Here's the drawing with two shaded views (mm, measured from the low corner). I have some questions. Round coordinates to 2 decimals unless told otherwise and drop trailing zeros. Loops run counter-clockwise (first coordinate to the right, second up) from the corner with the lowest first, then second, coordinate; pieces in that order, holes last.
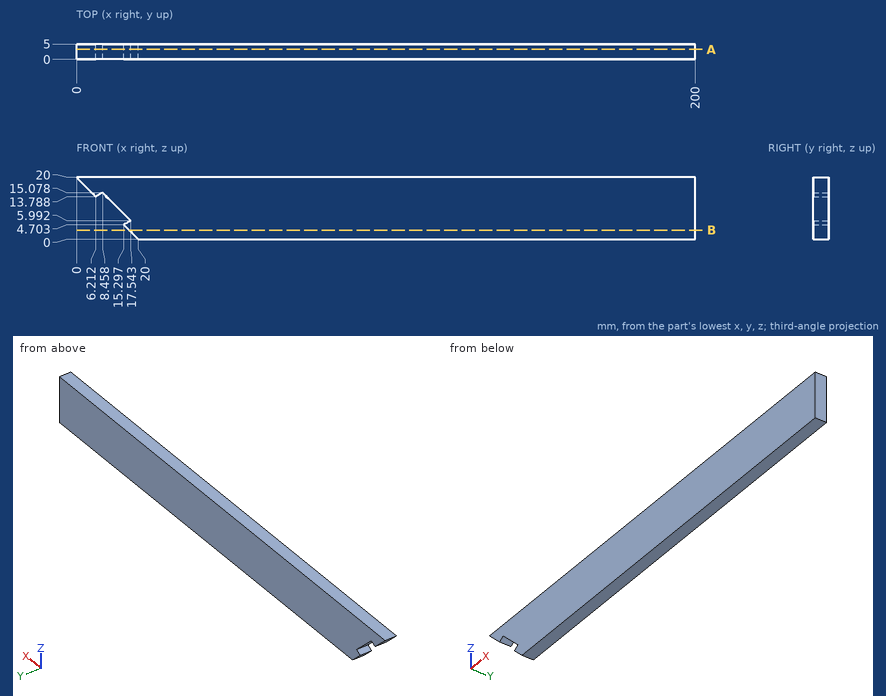
(1) If I drill on line 1 (Z direction, x = 9.5, y = 1.85) (1 decimal); line 2 (X direction, y = 4.3, z = 16.25); line 3 (X direction, y = 2.6, z = 2), over which ranges is the centre line in solid material (lowest first)?
Worked answers:
line 1: z = 14 to 20
line 2: x = 3.75 to 200
line 3: x = 18 to 200
(2) If we section it at B-B, the plane z = 3: List the corners of the cut face in (x, y) for me, then the cut area to 3 significant figures.
Worked answers:
outline: (17, 0) - (200, 0) - (200, 5) - (17, 5) - close
area: 915 mm2
(3) If we section it at A-A, the plane y = 3.25: List the corners of the cut face in (x, z) for me.
Worked answers:
outline: (0, 20) - (6.21, 13.79) - (8.46, 15.08) - (17.54, 5.99) - (15.3, 4.7) - (20, 0) - (200, 0) - (200, 20) - close
